```python
from build123d import *

# Parameters (mm, degrees)
SKETCH_1_W                = 100
SKETCH_1_H                = 157.5
EXTRUDE_1_DEPTH           = 18
SKETCH_2_W                = 90
SKETCH_2_H                = 220
CUT_EXTRUDE_1_DEPTH       = 2
SKETCH_3_W                = 90
SKETCH_3_H                = 195
CUT_EXTRUDE_2_DEPTH       = 2
SKETCH_4_W                = 60
SKETCH_4_H                = 8
EXTRUDE_2_DEPTH           = 100
EXTRUDE_3_DEPTH           = 6
HOLE_WIZARD_0_D           = 11
HOLE_WIZARD_0_CBORE_D     = 18
HOLE_WIZARD_0_CBORE_DEPTH = 11
HOLE_WIZARD_1_D           = 6.6
HOLE_WIZARD_1_CBORE_D     = 11
HOLE_WIZARD_1_CBORE_DEPTH = 6.8
FILLET_1_R                = 10
CUT_EXTRUDE_3_DEPTH       = 136.111296715
CHAMFER_1_SIZE            = 3
CHAMFER_2_SIZE            = 1


with BuildPart() as part:
    # 草图1 → 凸台-拉伸1 (new body)
    with BuildSketch(Plane.XY):
        Rectangle(SKETCH_1_W, SKETCH_1_H)
    extrude(amount=EXTRUDE_1_DEPTH)

    # 草图2 → 切除-拉伸1 (cut)
    with BuildSketch(Plane.XY.offset(18)):
        Rectangle(SKETCH_2_W, SKETCH_2_H)
    extrude(amount=-CUT_EXTRUDE_1_DEPTH, mode=Mode.SUBTRACT)

    # 草图3 → 切除-拉伸2 (cut)
    with BuildSketch(Plane.XY.offset(16)):
        with Locations((0, -78.75)):
            Rectangle(SKETCH_3_W, SKETCH_3_H)
    extrude(amount=-CUT_EXTRUDE_2_DEPTH, mode=Mode.SUBTRACT)

    # 草图4 → 凸台-拉伸2 (add)
    with BuildSketch(Plane.ZY.offset(50)):
        with Locations((-30, -27.5)):
            Rectangle(SKETCH_4_W, SKETCH_4_H)
    extrude(amount=-EXTRUDE_2_DEPTH)

    # 草图5 → 凸台-拉伸3 (add, symmetric)
    with BuildSketch(Plane(origin=(0, 0, 0), x_dir=(0, 0, -1), z_dir=(1, 0, 0))):
        Polygon((0, -31.5), (0, -78.75), (8, -78.75), (60, -39.5), (60, -31.5), align=None)
    extrude(amount=EXTRUDE_3_DEPTH, both=True)

    # 打孔尺寸(%根据)内六角圆柱头螺钉的类型0 (through all)
    with Locations(Plane(origin=(0, 0, 0), x_dir=(-1, 0, 0), z_dir=(0, 0, -1))):
        with Locations((-36, -1.5), (36, -1.5), (36, -53.5), (-36, -53.5)):
            CounterBoreHole(HOLE_WIZARD_0_D / 2, HOLE_WIZARD_0_CBORE_D / 2, HOLE_WIZARD_0_CBORE_DEPTH)

    # 打孔尺寸(%根据)内六角圆柱头螺钉的类型1 (through all)
    with Locations(Plane(origin=(0, 0, 0), x_dir=(-1, 0, 0), z_dir=(0, 0, -1))):
        with Locations((-14, 70.25), (-14, 42.25), (14, 70.25), (14, 42.25)):
            CounterBoreHole(HOLE_WIZARD_1_D / 2, HOLE_WIZARD_1_CBORE_D / 2, HOLE_WIZARD_1_CBORE_DEPTH)

    # 圆角1
    fillet_1_edges = [part.edges().sort_by_distance(p)[0] for p in [
        (0, -78.75, -8),
        (0, -39.5, -60),
    ]]
    fillet(fillet_1_edges, radius=FILLET_1_R)

    # 草图12 → 切除-拉伸3 (cut, through all)
    with BuildSketch(Plane.XZ.offset(31.5)):
        with BuildLine():
            Line((32.75, -42.5), (32.75, -47.5))
            ThreePointArc((32.75, -47.5), (30, -50.25), (27.25, -47.5))
            Line((27.25, -47.5), (27.25, -42.5))
            ThreePointArc((27.25, -42.5), (30, -39.75), (32.75, -42.5))
        make_face()
        with BuildLine():
            Line((32.75, -12.5), (32.75, -17.5))
            ThreePointArc((32.75, -17.5), (30, -20.25), (27.25, -17.5))
            Line((27.25, -17.5), (27.25, -12.5))
            ThreePointArc((27.25, -12.5), (30, -9.75), (32.75, -12.5))
        make_face()
        with BuildLine():
            Line((-32.75, -47.5), (-32.75, -42.5))
            ThreePointArc((-32.75, -42.5), (-30, -39.75), (-27.25, -42.5))
            Line((-27.25, -42.5), (-27.25, -47.5))
            ThreePointArc((-27.25, -47.5), (-30, -50.25), (-32.75, -47.5))
        make_face()
        with BuildLine():
            Line((-27.25, -12.5), (-27.25, -17.5))
            ThreePointArc((-27.25, -17.5), (-30, -20.25), (-32.75, -17.5))
            Line((-32.75, -17.5), (-32.75, -12.5))
            ThreePointArc((-32.75, -12.5), (-30, -9.75), (-27.25, -12.5))
        make_face()
    extrude(amount=-CUT_EXTRUDE_3_DEPTH, mode=Mode.SUBTRACT)

    # 倒角1
    chamfer_1_edges = [part.edges().sort_by_distance(p)[0] for p in [
        (-50, -27.5, -60),
        (50, -27.5, -60),
        (50, -78.75, 9),
        (-50, -78.75, 9),
        (-50, 78.75, 9),
        (50, 78.75, 9),
    ]]
    chamfer(chamfer_1_edges, length=CHAMFER_1_SIZE)

    # 倒角2
    chamfer_2_edges = [part.edges().sort_by_distance(p)[0] for p in [
        (-46, 78.75, 18),
        (46, -78.75, 18),
        (-45, 0, 18),
        (45, 0, 18),
        (-6, -59.616129225, -33.349331982),
        (6, -59.616129225, -33.349331982),
        (-6, -33.009585867, -60),
        (-6, -38.977573733, -58.951125718),
        (-6, -78.231967981, -7.826438724),
        (6, -33.009585867, -60),
        (6, -38.977573733, -58.951125718),
        (6, -78.231967981, -7.826438724),
        (0, 78.75, 16),
        (45, 78.75, 17),
        (45, -78.75, 16),
        (-45, 78.75, 17),
        (-45, -78.75, 16),
        (50, -53.625, 0),
        (50, -23.5, -28.5),
        (50, 0, 18),
        (0, -23.5, -60),
        (-48.5, -23.5, -58.5),
        (48.5, -23.5, -58.5),
        (26.5, -31.5, -60),
        (48.5, -31.5, -58.5),
        (-50, 26.125, 0),
        (-50, -31.5, -28.5),
        (-50, 0, 18),
        (-48.5, -31.5, -58.5),
        (-46, -78.75, 18),
        (-26.5, -78.75, 0),
        (-48.5, -77.25, 0),
        (-48.5, 77.25, 18),
        (-48.5, -77.25, 18),
        (48.5, -77.25, 0),
        (46, 78.75, 18),
        (48.5, 77.25, 18),
        (48.5, -77.25, 18),
        (0, 78.75, 0),
        (-48.5, 77.25, 0),
        (48.5, 77.25, 0),
        (0, -78.75, 14),
        (50, 26.125, 0),
        (-50, -53.625, 0),
        (-50, -23.5, -28.5),
        (50, -31.5, -28.5),
        (-26.5, -31.5, -60),
        (26.5, -78.75, 0),
        (-6, -78.75, -2.324801658),
        (6, -78.75, -2.324801658),
    ]]
    chamfer(chamfer_2_edges, length=CHAMFER_2_SIZE)


solid = part.part
```
Can you work these out from the model? Positions are in its coordinate system, mm. A direction names the side the tool comes from. Give positions to 0.01 mm unless a question says otherwise; leave off trailing zeros. Write item = value, one per line. Start each with the question number.
Q1. For faces 1 (the cylindrical face through (-30.06, -27.56, -39.75)), 2 (the flat face through (32, -49, 11)), 3 (the flat face through (-1, -78.75, 6)), 4 (the flat face through (6, -49, -23)), which set-ups out of +Z, -Z, +X, -X, +Y, -Y let a thin tool reach every point of the face, with its end or its side?
Q2. Suppose I cut it at A-A (x = 36). Count the separate pieces of the cut face and the enclosed holes in it, plus the area to 3 significant figures.
Q3. We'd pull the mould along X, two halves only. Please class faces 5 (the flat face through (48.172, 76.88, 17.493)), 6 (the cylindrical face through (13.57, 45.52, 11.46)), 7 (the cylindrical face through (-0.07, -38.92, -58.98)): pulls with the +X half, pulls with the -X half, needs draft (parallel to the pull), parting line crosses it, or undercut.
Q4. Will these pins go through, and if not, where does the flat tip stop? pin 1 Ø5 at (y, z) = (-47, -23.5) entering from +X; pin 2 Ø5.5 at (x, y) = (-34, 0.5) entering from -Z; pin 3 Ø6 at (x, z) = (38, -43) entering from -Y; pin 4 Ø5.5 at (x, y) = (14, 42.25) entering from -Z.
Q5. I need wall thicknesses on probe 1 along Y at (x, z) = (14, 4.25); probe 2 along X at (y, z) = (-53, 3); probe 3 along Y at (x, z) = (-36, 12). Which ranges of each line are inside material? Lowest first, please. Write a range as [from, to].
Check result:
q1.face_1 = +Y, -Y
q1.face_2 = -Z
q1.face_3 = +Z, -Z, +X, -X, -Y
q1.face_4 = -Z, +X, -Y
q2.separate_pieces = 3
q2.enclosed_holes = 0
q2.area = 2,340 mm2
q3.face_5 = pulls with the +X half
q3.face_6 = undercut
q3.face_7 = needs draft
q4.pin_1 = 6
q4.pin_2 = 11
q4.pin_3 = -31.5
q4.pin_4 = through
q5.probe_1 = [-78.75, 36.75], [47.75, 64.75], [75.75, 78.75]
q5.probe_2 = [-50, -44.99], [-27.01, 27.01], [44.99, 50]
q5.probe_3 = [-78.75, -59], [-48, -7], [4, 78.75]
